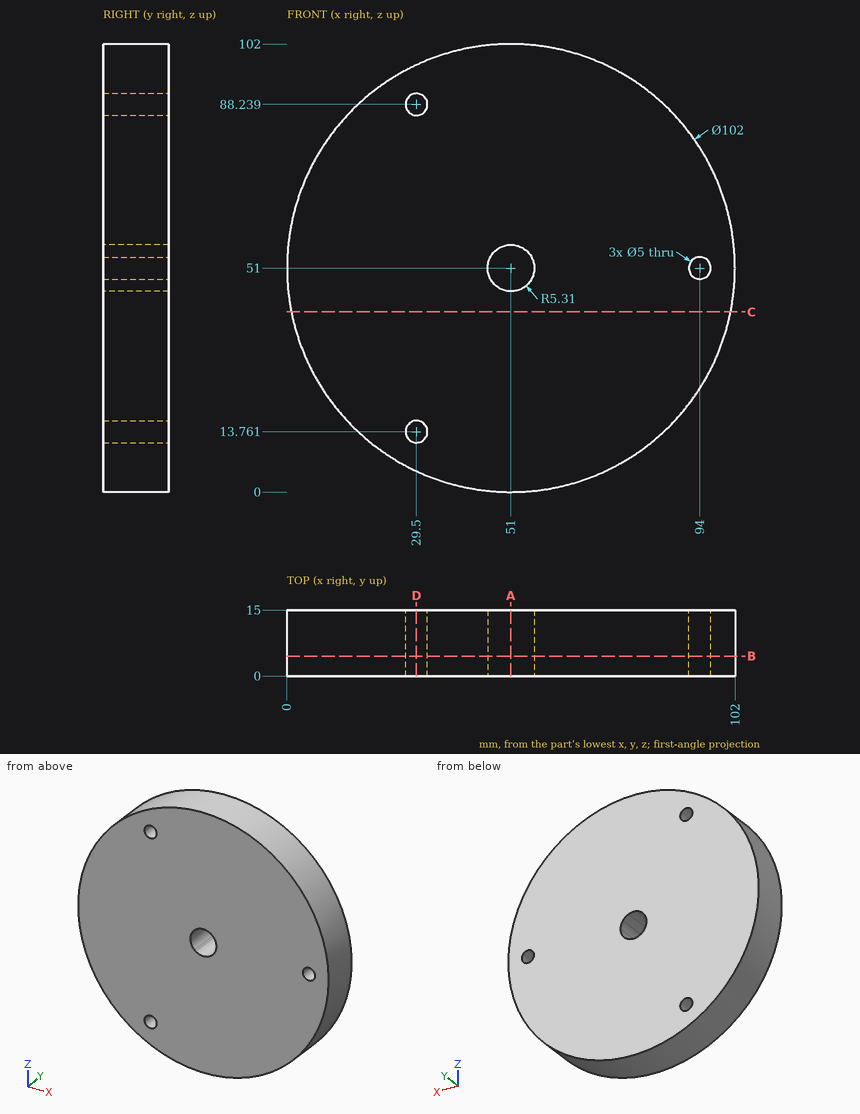
Source: three-view drawing plus pictorial views. Frame: mm from the lowest corner of the part. Round coordinates to 2 decimals unless told otherwise and drop trailing zeros. Loops run counter-clockwise (first coordinate to the right, second up) from the corner with the lowest first, then second, coordinate; pieces in that order, holes last.
Q1. Material intervals for L1, parallel to Z at x = 29.5, y = 3.5; L2, parallel to X at y = 10.5, z = 53; L3, parallel to Z at x = 95, y = 10.75, sorted ascending.
Q2. Section D-D on x = 29.5. Return loops of the section in (y, z), plus the area to 3 significant figures.
Q3. Section B-B on y = 4.5. Return loops of the section in (x, z) (1 decimal).
Q4. Section C-C on z = 41. Return loops of the section in (x, y), plus the area to 3 significant figures.
Q5. Section A-A on x = 51. Return loops of the section in (y, z), plus the area to 3 significant figures.
Q6. Pin query (flat end, axial travel): P1, Ø2, axis at y = 8, z = 89, coming from the +X side; P2, Ø4, axis at x = 29.5, z = 13.76, coming from the +Y side; P3, Ø6, axis at x = 29.5, y = 7, coming from the -Z side; P4, Ø1, axis at x = 21.5, y = 5.5, coming from the -Z side. Return the tip coordinate at first contact, or that it passes through.
Evaluation:
1. L1: z = 4.75 to 11.26, 16.26 to 85.74, 90.74 to 97.25
1. L2: x = 0.04 to 46.08, 55.92 to 92.5, 95.5 to 101.96
1. L3: z = 25.21 to 48.71, 53.29 to 76.79
2. outline: (0, 4.75) - (15, 4.75) - (15, 11.26) - (0, 11.26) - close; (0, 16.26) - (15, 16.26) - (15, 85.74) - (0, 85.74) - close; (0, 90.74) - (15, 90.74) - (15, 97.25) - (0, 97.25) - close
2. area: 1,240 mm2
3. outline: circle Ø102 at (51, 51); hole circle Ø5 at (29.5, 13.8); hole circle Ø5 at (29.5, 88.2); hole (45.9, 52.3) arc R5.3 ccw to (47.4, 47.1) arc R5.3 ccw to (47.9, 46.7) arc R5.3 ccw to (53.3, 46.2) arc R5.3 ccw to (55.4, 48) arc R5.3 ccw to (56.3, 51) arc R5.3 ccw to (55.4, 54) arc R5.3 ccw to (53, 55.9) arc R5.3 ccw to (47.2, 54.7) arc R5.3 ccw to start; hole circle Ø5 at (94, 51)
4. outline: (0.99, 0) - (101.01, 0) - (101.01, 15) - (0.99, 15) - close
4. area: 1,500 mm2
5. outline: (0, 0) - (15, 0) - (15, 45.69) - (0, 45.69) - close; (0, 56.31) - (15, 56.31) - (15, 102) - (0, 102) - close
5. area: 1,370 mm2
6. P1: stops at x = 86.1
6. P2: passes through
6. P3: stops at z = 3.47
6. P4: stops at z = 9.05
